Geometry check sheet. Reference: drawing and pictorial views, mm from the part's lowest x, y, z. A direction names the side the tool comes from. Round coordinates to 2 decimals unless told otherwise and drop trailing zeros. Loops run counter-clockwise (first coordinate to the right, second up) from the corner with the lowest first, then second, coordinate; pieces in that order, holes last. Notation, with made-up numbers: (-24, 18.25) -> (33, 18.25) arc R26 cw to (33, 38.25) -> close; hole circle Ø6 at (51, 19.25). An arc over 180 degrees is marked (long way). Write item = value, one per line.
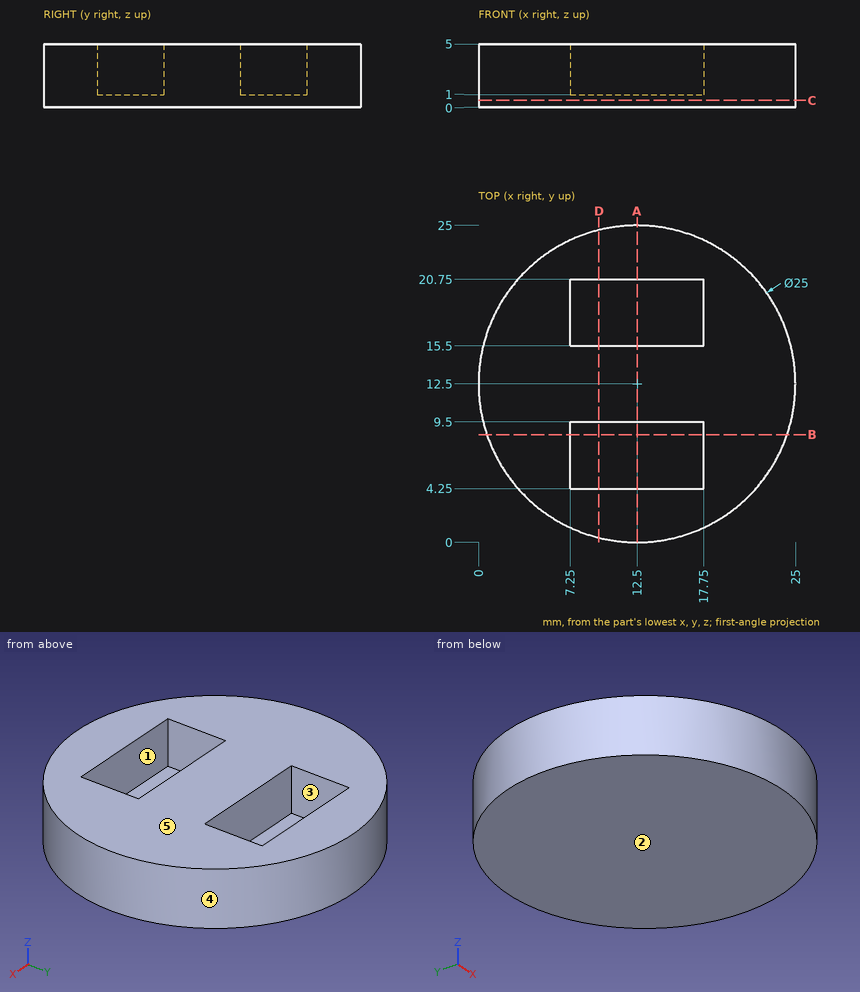
(1) Sectioned sample at A-A, the plane x = 12.5. Record the cut outline in (y, z).
Filled sheet:
outline = (0, 0) -> (25, 0) -> (25, 5) -> (20.75, 5) -> (20.75, 1) -> (15.5, 1) -> (15.5, 5) -> (9.5, 5) -> (9.5, 1) -> (4.25, 1) -> (4.25, 5) -> (0, 5) -> close
(2) Sectioned sample at C-C, the plane z = 0.55. Record the cut outline in (x, y), and give its area (3 significant figures).
Filled sheet:
outline = circle Ø25 at (12.5, 12.5)
area = 491 mm2
(3) Draft check along Y on the marked faces 3, 4 and 5. Enter one of: released by +Y, released by -Y, zero draft, split by the parting line, or undercut.
Filled sheet:
face_3 = undercut
face_4 = split by the parting line
face_5 = zero draft
(4) Sectioned sample at D-D, the plane x = 9.5. Record the cut outline in (y, z).
Filled sheet:
outline = (0.37, 0) -> (24.63, 0) -> (24.63, 5) -> (20.75, 5) -> (20.75, 1) -> (15.5, 1) -> (15.5, 5) -> (9.5, 5) -> (9.5, 1) -> (4.25, 1) -> (4.25, 5) -> (0.37, 5) -> close
(5) Set-up check for the marked faces 1 and 2: record each of +Z, -Z, +X, -X, +Y, -Y from which the full face is reachable in a straight line by a thin tool's end or side.
Filled sheet:
face_1 = +Z
face_2 = -Z, +X, -X, +Y, -Y
(6) Material ranges on probe 1 along Y at (x, z) = (15, 3.7); probe 2 along Y at (x, z) = (10.75, 1.1); probe 3 along X at (y, z) = (4.75, 3.9), recorded low to high. Write a range as from..to.
Filled sheet:
probe_1 = 0.25..4.25, 9.5..15.5, 20.75..24.75
probe_2 = 0.12..4.25, 9.5..15.5, 20.75..24.88
probe_3 = 2.69..7.25, 17.75..22.31
(7) Go/stop test with flat-tipped pins: pin 1 Ø1.5 at (y, z) = (14, 2) entering from +X; pin 2 Ø1.6 at (x, y) = (13.5, 7) entering from +Z; pin 3 Ø3 at (x, z) = (10.5, 2.5) entering from -Y. Record where each tip stops, or that it passes through.
Filled sheet:
pin_1 = 24.98
pin_2 = 1
pin_3 = 0.01
(8) Sectioned sample at B-B, the plane y = 8.5. Record the cut outline in (x, z), and give its area (3 significant figures).
Filled sheet:
outline = (0.66, 0) -> (24.34, 0) -> (24.34, 5) -> (17.75, 5) -> (17.75, 1) -> (7.25, 1) -> (7.25, 5) -> (0.66, 5) -> close
area = 76.4 mm2
